Build history of the part. All positions in model axes, mm. A direction names the side the tool comes from. Round coordinates to 2 decimals unless told otherwise and drop trailing zeros. Loops run counter-clockwise (first coordinate to the right, second up) from the corner with the lowest first, then second, coordinate; pieces in that order, holes last.
from build123d import *

# Parameters (mm, degrees)
BOSS_EXTRUDE1_DEPTH = 5.842
SKETCH2_R           = 3.175
CUT_EXTRUDE1_DEPTH  = 33.78403476
CUT_EXTRUDE3_DEPTH  = 33.78403476
SKETCH5_W           = 50.8
SKETCH5_H           = 1.5875
BOSS_EXTRUDE2_DEPTH = 5.842


with BuildPart() as part:
    # Sketch1 → Boss-Extrude1 (new body)
    with BuildSketch(Plane(origin=(0, 0, 0), x_dir=(1, 0, 0), z_dir=(0, 1, 0))):
        Polygon((31.242, -6.450000054), (25.4, -6.450000054), (25.4, -7.837499946), (-25.4, -7.837499946), (-25.4, -6.450000054), (-31.242, -6.450000054), (-31.242, 6.450000054), (-25.4, 6.450000054), (-25.4, 8.037500054), (25.4, 8.037500054), (25.4, 6.450000054), (31.242, 6.450000054), align=None)
    extrude(amount=BOSS_EXTRUDE1_DEPTH)

    # Sketch2 → Cut-Extrude1 (cut, through all)
    with BuildSketch(Plane(origin=(0, 5.842, 0), x_dir=(1, 0, 0), z_dir=(0, 1, 0))):
        with Locations(Location((-19.05, 0, 0), (0, 0, 270))):
            Circle(SKETCH2_R)
        with Locations(Location((19.05, 0, 0), (0, 0, 90))):
            Circle(SKETCH2_R)
    extrude(amount=-CUT_EXTRUDE1_DEPTH, mode=Mode.SUBTRACT)

    # Sketch4 → Cut-Extrude3 (cut, through all)
    with BuildSketch(Plane(origin=(0, 0, 0), x_dir=(-1, 0, 0), z_dir=(0, -1, 0))):
        with BuildLine():
            Line((3.175, -3.074999946), (3.175, 3.275000054))
            ThreePointArc((3.175, 3.275000054), (4.7625, 4.862500054), (6.35, 3.275000054))
            Line((6.35, 3.275000054), (6.35, -3.074999946))
            ThreePointArc((6.35, -3.074999946), (4.7625, -4.662499946), (3.175, -3.074999946))
        make_face()
        with BuildLine():
            Line((-3.175, -3.074999946), (-3.175, 3.275000054))
            ThreePointArc((-3.175, 3.275000054), (-4.7625, 4.862500054), (-6.35, 3.275000054))
            Line((-6.35, 3.275000054), (-6.35, -3.074999946))
            ThreePointArc((-6.35, -3.074999946), (-4.7625, -4.662499946), (-3.175, -3.074999946))
        make_face()
    extrude(amount=-CUT_EXTRUDE3_DEPTH, mode=Mode.SUBTRACT)

    # Sketch5 → Boss-Extrude2 (add)
    with BuildSketch(Plane(origin=(0, 0, 0), x_dir=(-1, 0, 0), z_dir=(0, -1, 0))):
        with Locations((0, 8.831250054)):
            Rectangle(SKETCH5_W, SKETCH5_H)
    extrude(amount=-BOSS_EXTRUDE2_DEPTH)


solid = part.part
(1) Pull direction Z, two halves, no side cores. Call faces 1 (the face through (4.797, 2.88, 4.662)), 2 (the face through (31.242, 3, 0)), 3 (the face through (28, 3, -6.45)): +Z half, -Z half, draft (parallel to the pull), parting line (faces both ways), or undercut.
Responses:
face 1: undercut
face 2: draft
face 3: -Z half
(2) Slice it at B-B on x = -19.05. List the corners of the cut face in (y, z) (1 decimal), plus the area to 3 significant figures.
Responses:
outline: (0, -9.6) - (5.8, -9.6) - (5.8, -3.2) - (0, -3.2) - close; (0, 3.2) - (5.8, 3.2) - (5.8, 7.8) - (0, 7.8) - close
area: 64.9 mm2
(3) Pin check, flat tips, straight feed: P1, Ø1, axis at y = 3.5, z = -8.5, coming from the +X side; P2, Ø1.8, axis at x = 29, y = 4, coming from the +Z side; P3, Ø1.8, axis at x = -28.5, y = 2.5, coming from the -Z side. Stop position of each tip, or through.
Responses:
P1: stops at x = 25.4
P2: stops at z = 6.45
P3: stops at z = -6.45
(4) Which spindle directions (+Z, -Z, +X, -X, +Y, -Y) get a long thin tool onto all of the face, cutting with end or side? Do faces 4 (the face through (28, 3, 6.45)), 5 (the face through (-25.4, 3, -8)), 6 (the face through (25.4, 3, -8)), 7 (the face through (-4.797, 2.88, 4.662)). Say none if no direction does.
Responses:
face 4: +Z, +X, +Y, -Y
face 5: -Z, -X, +Y, -Y
face 6: -Z, +X, +Y, -Y
face 7: +Y, -Y
(5) Slice it at A-A on z = 0. List the corners of the cut face in (x, y) (3 decimals), plus the area to 3 significant figures.
Responses:
outline: (-31.242, 0) - (-22.225, 0) - (-22.225, 5.842) - (-31.242, 5.842) - close; (-15.875, 0) - (-6.35, 0) - (-6.35, 5.842) - (-15.875, 5.842) - close; (-3.175, 0) - (3.175, 0) - (3.175, 5.842) - (-3.175, 5.842) - close; (6.35, 0) - (15.875, 0) - (15.875, 5.842) - (6.35, 5.842) - close; (22.225, 0) - (31.242, 0) - (31.242, 5.842) - (22.225, 5.842) - close
area: 254 mm2
(6) Slice it at C-C on y = 0.85. Count the separate pieces of the cut face and the enclosed holes in it, plus the area to 3 significant figures.
Responses:
separate pieces: 1
enclosed holes: 4
area: 918 mm2
(7) Probe line 1 (X direction, y = 3.7, z = 0) (3 decimals); line 2 (Z direction, x = 19.05, y = 2.45) (1 decimal); line 3 (X direction, y = 1.55, z = -7.75). List the from-to ranges inside material, lowest first.
Responses:
line 1: x = -31.242 to -22.225, -15.875 to -6.35, -3.175 to 3.175, 6.35 to 15.875, 22.225 to 31.242
line 2: z = -9.6 to -3.2, 3.2 to 7.8
line 3: x = -25.4 to 25.4
(8) Slice it at D-D on z = -2.5. List the corners of the cut face in (x, y) (3 decimals).
Responses:
outline: (-31.242, 0) - (-21.007, 0) - (-21.007, 5.842) - (-31.242, 5.842) - close; (-17.093, 0) - (-6.35, 0) - (-6.35, 5.842) - (-17.093, 5.842) - close; (-3.175, 0) - (3.175, 0) - (3.175, 5.842) - (-3.175, 5.842) - close; (6.35, 0) - (17.093, 0) - (17.093, 5.842) - (6.35, 5.842) - close; (21.007, 0) - (31.242, 0) - (31.242, 5.842) - (21.007, 5.842) - close
